```python
from build123d import *

# Parameters (mm, degrees)
F1_DEPTH = 6
F2_R     = 18
F2_R_2   = 12.5
F3_DEPTH = 25


with BuildPart() as f1:
    # F0 (on Right) → F1 (new body)
    with BuildSketch(Plane.YZ):
        Polygon((61.581665, 58.027008), (-256.018335, 58.027008), (-262.018335, 58.027008), (-262.018335, 33.027008), (-256.018335, 33.027008), (-256.018335, -16.972992), (-262.018335, -16.972992), (-262.018335, -41.972992), (-256.018335, -41.972992), (61.581665, -41.972992), (67.581665, -41.972992), (67.581665, -16.972992), (61.581665, -16.972992), (61.581665, 33.027008), (67.581665, 33.027008), (67.581665, 58.027008), align=None)
    extrude(amount=F1_DEPTH)

    # F2 (on face) → F3 (cut)
    with BuildSketch(Plane.YZ.offset(6)):
        with Locations((-179.618335, 8.027008)):
            Circle(F2_R)
        with Locations((-97.218335, 8.027008)):
            Circle(F2_R_2)
        with Locations((-14.818335, 8.027008)):
            Circle(F2_R)
    extrude(amount=-F3_DEPTH, mode=Mode.SUBTRACT)


solid = f1.part
```
Input: part model. Units: mm. Frame: model coordinates. A direction names the side the tool comes from. Give positions to 0.01 mm unless a question says otherwise; leave off trailing zeros. Loops run counter-clockwise (first coordinate to the right, second up) from the corner with the lowest first, then second, coordinate; pieces in that order, holes last.
1) Section query C-C on x = 1.3. Return the cut outline in (y, z).
A:
outline: (-262.02, -41.97) - (67.58, -41.97) - (67.58, -16.97) - (61.58, -16.97) - (61.58, 33.03) - (67.58, 33.03) - (67.58, 58.03) - (-262.02, 58.03) - (-262.02, 33.03) - (-256.02, 33.03) - (-256.02, -16.97) - (-262.02, -16.97) - close; hole circle Ø36 at (-179.62, 8.03); hole circle Ø25 at (-97.22, 8.03); hole circle Ø36 at (-14.82, 8.03)
2) Section query D-D on y = -104. Return the cut outline in (x, z), and give its area (3 significant figures).
A:
outline: (0, -41.97) - (6, -41.97) - (6, -2.47) - (0, -2.47) - close; (0, 18.53) - (6, 18.53) - (6, 58.03) - (0, 58.03) - close
area: 474 mm2
3) Mould query, pull axis Y, two halves, no side actions, for faces 4 (the cylindrical face through (3.04, 1.81, 1.13)), 5 (the flat face through (3, -100, -41.973)), 6 (the flat face through (3, -262.018, -29)). Classes: released by +Y, released by -Y, zero draft, split by the parting line, or undercut.
A:
face 4: undercut
face 5: zero draft
face 6: released by -Y
4) Section query A-A on z = 13.5. Return the cut outline in (x, y), and give its area (3 significant figures).
A:
outline: (0, -256.02) - (6, -256.02) - (6, -196.77) - (0, -196.77) - close; (0, -162.47) - (6, -162.47) - (6, -108.46) - (0, -108.46) - close; (0, -85.98) - (6, -85.98) - (6, -31.97) - (0, -31.97) - close; (0, 2.33) - (6, 2.33) - (6, 61.58) - (0, 61.58) - close
area: 1,360 mm2
5) Reachability of faces 1 (the flat face through (3, -256.018, 8)), 2 (the flat face through (3, 67.582, 45)), 3 (the flat face through (3, 65, 33.027)) from +Z, -Z, +X, -X, +Y, -Y: full face, straight path, thin tool, end or side. Return the list, or none.
A:
face 1: +X, -X, -Y
face 2: +Z, -Z, +X, -X, +Y
face 3: +X, -X, +Y
6) Section query B-B on y = -165. Return the cut outline in (x, z), and give its area (3 significant figures).
A:
outline: (0, -41.97) - (6, -41.97) - (6, -2.48) - (0, -2.48) - close; (0, 18.53) - (6, 18.53) - (6, 58.03) - (0, 58.03) - close
area: 474 mm2
7) Contact query for flat-ended pins moving along their axis: pin 1 (3 mm diameter, centred on x = 4, z = 19.5, fed in from -Y); pin 2 (6 mm diameter, centred on y = -45, z = 38.5, fed in from -X). Output: stop coordinate, or through.
A:
pin 1: stops at y = -256.02
pin 2: stops at x = 0
8) Line query: L1, parallel to Y at x = 2.95, z = 22.5; L2, parallel to Y at x = 1.7, z = -1.5; L3, parallel to Y at x = 2.45, z = 28. Output: solid intervals per line, ascending.
A:
L1: y = -256.02 to -190.32, -168.92 to -25.52, -4.12 to 61.58
L2: y = -256.02 to -194.89, -164.35 to -105.31, -89.13 to -30.09, 0.45 to 61.58
L3: y = -256.02 to 61.58
